```python
from build123d import *

# Parameters (mm, degrees)
SKETCH1_W           = 122
SKETCH1_H           = 99
BOSS_EXTRUDE1_DEPTH = 48
SKETCH2_W           = 114
SKETCH2_H           = 91
CUT_EXTRUDE1_DEPTH  = 44
SKETCH3_R           = 2
CUT_EXTRUDE2_DEPTH  = 141.13654056


with BuildPart() as part:
    # Sketch1 → Boss-Extrude1 (new body)
    with BuildSketch(Plane(origin=(0, 0, 0), x_dir=(1, 0, 0), z_dir=(0, 1, 0))):
        Rectangle(SKETCH1_W, SKETCH1_H)
    extrude(amount=BOSS_EXTRUDE1_DEPTH)

    # Sketch2 → Cut-Extrude1 (cut)
    with BuildSketch(Plane(origin=(0, 48, 0), x_dir=(1, 0, 0), z_dir=(0, 1, 0))):
        Rectangle(SKETCH2_W, SKETCH2_H)
    extrude(amount=-CUT_EXTRUDE1_DEPTH, mode=Mode.SUBTRACT)

    # Sketch3 → Cut-Extrude2 (cut, through all)
    with BuildSketch(Plane(origin=(61, 0, 0), x_dir=(0, 0, -1), z_dir=(1, 0, 0))):
        with Locations((-19.5, 24)):
            Circle(SKETCH3_R)
        with Locations((5.5, 24)):
            Circle(SKETCH3_R)
    extrude(amount=-CUT_EXTRUDE2_DEPTH, mode=Mode.SUBTRACT)


solid = part.part
```
Input: part model. Units: mm. Frame: model coordinates. A direction names the side the tool comes from. Round coordinates to 2 decimals unless told otherwise and drop trailing zeros. Loops run counter-clockwise (first coordinate to the right, second up) from the corner with the lowest first, then second, coordinate; pieces in that order, holes last. Notation, with made-up numbers: M 59,5 L 70,5 A13 ccw 70,24 Z; hole C -14.75,2.5 d8. An arc over 180 degrees is marked long. Answer in a Markdown table with one row per item. Add a question column.
1. Section B-B (y = 32). Output: boundary loops of the cut face in (x, z), and give its area (3 significant figures).
2. Mould query, pull axis Z, two halves, no side actions, for faces 1 (the face through (61, 24, 1)), 2 (the face through (-1, 4, -1)), 3 (the face through (-1, 24, -49.5)). Classes: released by +Z, released by -Z, zero draft, split by the parting line, or undercut.
3. Section D-D (y = 24). Output: boundary loops of the cut face in (x, z), and give its area (3 significant figures).
4. Ray query, probe 1 along X at (y, z) = (30, -3); probe 2 along Z at (x, y) = (37.5, 28); probe 3 along Y at (x, z) = (-58, -5.5). Return the intervals inside material, ascending.
5. Set-up query: faces 4 (the face through (59, 22.8, -3.9)), 5 (the face through (-57, 26, 1)). Return all of +Z, -Z, +X, -X, +Y, -Y with unobstructed straight access to the full face (end or side cutting, diameter ignored); none if empty.
6. Section A-A (z = 19.5). Output: boundary loops of the cut face in (x, y), and give its area (3 significant figures).
7. Section C-C (x = -41.5). Output: boundary loops of the cut face in (y, z), and give its area (3 significant figures).
8. Contact query for a flat-ended pin moving along its axis: pin 1 (2.5 mm diameter, centred on y = 24, z = -5.5, fed in from +X). Output: stop coordinate, or through.
Values follow:
| question | item | result |
|---|---|---|
| 1 | outline | M -61,-49.5 L 61,-49.5 L 61,49.5 L -61,49.5 Z; hole M -57,-45.5 L 57,-45.5 L 57,45.5 L -57,45.5 Z |
| 1 | area | 1,700 mm^2 |
| 2 | face 1 | zero draft |
| 2 | face 2 | undercut |
| 2 | face 3 | released by -Z |
| 3 | outline | M -61,-49.5 L 61,-49.5 L 61,-7.5 L 57,-7.5 L 57,-45.5 L -57,-45.5 L -57,-7.5 L -61,-7.5 Z; M -61,-3.5 L -57,-3.5 L -57,17.5 L -61,17.5 Z; M -61,21.5 L -57,21.5 L -57,45.5 L 57,45.5 L 57,21.5 L 61,21.5 L 61,49.5 L -61,49.5 Z; M 57,-3.5 L 61,-3.5 L 61,17.5 L 57,17.5 Z |
| 3 | area | 1,640 mm^2 |
| 4 | probe 1 | -61 to -57, 57 to 61 |
| 4 | probe 2 | -49.5 to -45.5, 45.5 to 49.5 |
| 4 | probe 3 | 0 to 22, 26 to 48 |
| 5 | face 4 | +X, -X |
| 5 | face 5 | +Y |
| 6 | outline | M -61,0 L 61,0 L 61,22 L 57,22 L 57,4 L -57,4 L -57,22 L -61,22 Z; M -61,26 L -57,26 L -57,48 L -61,48 Z; M 57,26 L 61,26 L 61,48 L 57,48 Z |
| 6 | area | 808 mm^2 |
| 7 | outline | M 0,-49.5 L 48,-49.5 L 48,-45.5 L 4,-45.5 L 4,45.5 L 48,45.5 L 48,49.5 L 0,49.5 Z |
| 7 | area | 748 mm^2 |
| 8 | pin 1 | through |
